Verification items for the finished model (mm, model axes). A direction names the side the tool comes from. Round coordinates to 2 decimals unless told otherwise and drop trailing zeros. Order: outer loops, then holes, each group sorted by start corner. A loop starts at its lowest first (then second) coordinate and runs counter-clockwise, first axis right, second up. Notation, with made-up numbers: (54, -28.5) -> (63, -28.5) arc R20 cw to (63, 0.5) -> close; hole circle Ø2 at (81, 22). An arc over 180 degrees is marked (long way). Put each result on its own line as item: value.
```python
from build123d import *

# Parameters (mm, degrees)
F2_R     = 0.9
F3_DEPTH = 8


with BuildPart() as f1:
    # F0 (on Right) → F1 (revolve)
    with BuildSketch(Plane.YZ):
        with BuildLine():
            Line((0, 5.841069423), (0, 0))
            Line((0, 0), (12, 0))
            Line((12, 0), (12, 2))
            add(Edge.make_bspline(
                [(0, 5.841069423), (0.3497183744, 5.8426503833), (1.3005439266, 5.8382623264), (2.8964802159, 5.7455783673), (4.5870476785, 5.3782777015), (5.9874523646, 4.7970685822), (7.0213600835, 4.1135251272), (7.9242720145, 3.365273981), (8.9405324509, 2.6085376072), (10.1254552113, 2.0890201928), (11.1979079035, 1.9926198646), (11.7889157433, 1.9938020422), (12, 2)],
                knots=[0.0080728178, 0.0080728178, 0.0080728178, 0.0080728178, 1.0595032706, 2.8567052188, 4.7969778976, 6.2186626182, 7.3787538627, 8.5000771421, 9.7368937359, 11.1749138539, 12.3063283312, 12.9431817135, 12.9431817135, 12.9431817135, 12.9431817135], degree=3))
        make_face()
        with BuildLine():
            Line((0, 6.841), (0, 5.841069423))
            add(Edge.make_bspline(
                [(0, 5.841069423), (0.3497183744, 5.8426503833), (1.3005439266, 5.8382623264), (2.8964802159, 5.7455783673), (4.5870476785, 5.3782777015), (5.9874523646, 4.7970685822), (7.0213600835, 4.1135251272), (7.9242720145, 3.365273981), (8.9405324509, 2.6085376072), (10.1254552113, 2.0890201928), (11.1979079035, 1.9926198646), (11.7889157433, 1.9938020422), (12, 2)],
                knots=[0.0080728178, 0.0080728178, 0.0080728178, 0.0080728178, 1.0595032706, 2.8567052188, 4.7969778976, 6.2186626182, 7.3787538627, 8.5000771421, 9.7368937359, 11.1749138539, 12.3063283312, 12.9431817135, 12.9431817135, 12.9431817135, 12.9431817135], degree=3))
            Line((12, 2), (38.25, 2))
            Line((38.25, 2), (38.25, 3))
            Line((38.25, 3), (12, 3))
            add(Edge.make_bspline(
                [(0, 6.841), (8.7633541102, 6.7704077573), (7.4586680881, 3), (12, 3)],
                knots=[0, 0, 0, 0, 12.5997333702, 12.5997333702, 12.5997333702, 12.5997333702], degree=3))
        make_face()
    revolve(axis=Axis((0, 19.125, 0), (0, -1, 0)))

    # F2 (on face) → F3 (cut)
    with BuildSketch(Plane.XZ):
        Circle(F2_R)
    extrude(amount=-F3_DEPTH, mode=Mode.SUBTRACT)

    # F4: F1 across face


with BuildPart() as f1_1:
    add(f1.part)
    add(f1.part.mirror(Plane(origin=(0, 38.25, 0), x_dir=(-1, 0, 0), z_dir=(0, 1, 0))))


solid = f1_1.part
```
Item 1: Sectioned sample at A-A, the plane y = 58. Record the boundary of the cut face in (x, z).
Geometry check:
outline: circle Ø6 at (0, 0); hole circle Ø4 at (0, 0)
Item 2: Depth check by flat-ended pin: pin 1 Ø5 at (x, y) = (1, 10) entering from -Z; pin 2 Ø8 at (x, y) = (-4.5, 31) entering from +Z. Enter the tip coordinate at first touch or a pass-through.
Geometry check:
pin 1: z = -4.89
pin 2: z = 2.96
Item 3: Release check for a two-part mould opening along Z. For faces 1 (the face through (0, 64.5, 0)), 2 (the face through (1.4, 76.5, -0.1)), 3 (the face through (0, 39, -3)) record: pulls with the +Z half, pulls with the -Z half, needs draft (parallel to the pull), parting line crosses it, or undercut.
Geometry check:
face 1: undercut
face 2: needs draft
face 3: parting line crosses it
Item 4: Tool access check on faces 4 (the face through (0.86, 72.56, 0.27)), 5 (the face through (0, 8, 0)), 6 (the face through (0, 12, 0)). Record the directions out of +Z, -Z, +X, -X, +Y, -Y that give a thin tool (end or side, any length) a straight path to the whole face; none if there is none.
Geometry check:
face 4: +Y
face 5: -Y
face 6: none
Item 5: Material ranges on line 1 along X through (y, z) = (57.5, 0); line 2 along Z through (x, y) = (-0.25, 35); line 3 along X through (y, z) = (58.5, -2.25), recorded low to high.
Geometry check:
line 1: -3 to -2, 2 to 3
line 2: -2.99 to -1.98, 1.98 to 2.99
line 3: -1.98 to 1.98
